Geometry: final body of the model. Coordinates: model frame, mm. Face numbers are marked on the shaded views. A direction names the side the tool comes from. Give positions to 0.01 mm unless a question says otherwise; leave off trailing zeros. Write each loop counter-clockwise with the first axis right and the second up, starting at its lowest first coordinate (ties: lowest second). Pieces come first, ordered by that corner, then holes. Notation, with made-up numbers: (9, 13.5) -> (36, 13.5) arc R30 cw to (36, 50.5) -> close; hole circle Ø5 at (77, 6). An arc over 180 degrees is marked (long way). Answer as a JSON object with one key per item and string values.
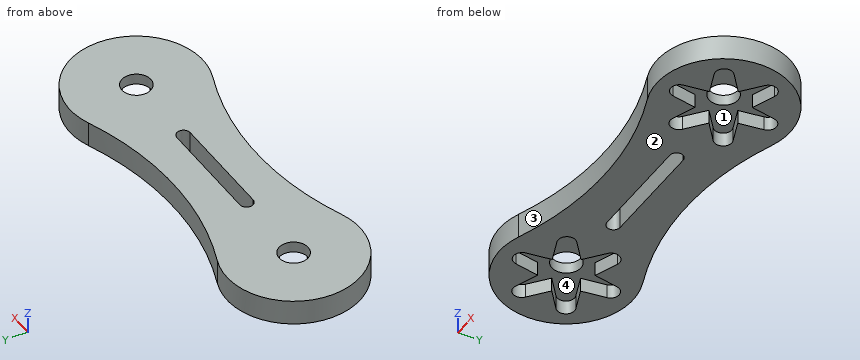
Autodesk Inventor part; units mm, degrees
ref_plane "Work Plane2" through (-40, 0, 7.55) normal (-1, 0, 0) x (0, -1, 0)
ref_plane "YZ Plane" through (0, 0, 0) normal (1, 0, 0) x (0, 1, 0)
ref_plane "XZ Plane" through (0, 0, 0) normal (0, 1, 0) x (-1, 0, 0)
sketch "Sketch1" plane through (0, 0, 0) normal (0, 0, 1) x (1, 0, 0)
  arc A0 (-72.7273, 18.6308) -> (-72.7273, -18.6308) centre (-80, 0) ccw
  arc A1 (-7.2727, -18.6308) -> (-72.7273, -18.6308) centre (-40, -102.4695) ccw
  arc A2 (-7.2727, -18.6308) -> (-7.2727, 18.6308) centre (0, 0) ccw
  arc A3 (-72.7273, 18.6308) -> (-7.2727, 18.6308) centre (-40, 102.4695) ccw
  arc A4 (-79.5765, 3.9775) -> (-79.5765, -3.9775) centre (-80, 0) ccw
  arc A5 (-0.4235, -3.9775) -> (-0.4235, 3.9775) centre (0, 0) ccw
  arc A6 (-80.4235, -3.9775) -> (-80.4235, 3.9775) centre (-80, 0) ccw
  arc A7 (-0.4235, 3.9775) -> (-0.4235, -3.9775) centre (0, 0) ccw
  point P0 (-103.8261, -115.9088)
  dimension "d0" = 20
  dimension "d1" = 20
  dimension "d2" = 90
  dimension "d3" = 90
  dimension "d4" = 4
  dimension "d7" = 80
  dimension "d33" = 4
extrude "Extrusion1" add sketch "Sketch1" along normal blind 7.55 contours A3 A2 A1 A0 | A6 A4 | A7 A5
sketch "Sketch3" plane through (0, 0, 7.55) normal (0, 0, 1) x (1, 0, 0)
  arc A0 (-72.7273, 18.6308) -> (-72.7273, -18.6308) centre (-80, 0) ccw
  arc A1 (-7.2727, -18.6308) -> (-72.7273, -18.6308) centre (-40, -102.4695) ccw
  arc A2 (-7.2727, -18.6308) -> (-7.2727, 18.6308) centre (0, 0) ccw
  arc A3 (-72.7273, 18.6308) -> (-7.2727, 18.6308) centre (-40, 102.4695) ccw
  line L0 (-56.02, 2) -> (-23.98, 2)
  line L1 (-56.02, -2) -> (-23.98, -2)
  arc A4 (-56.02, 2) -> (-56.02, -2) centre (-56.02, 0) ccw
  arc A5 (-23.98, -2) -> (-23.98, 2) centre (-23.98, 0) ccw
  point P0 (-83.48, 0)
  dimension "d12" = 2
extrude "Extrusion2" cut sketch "Sketch3" against normal blind 10 contours L0 A5 L1 A4
ref_plane "Work Plane2" through (-40, 0, 7.55) normal (-1, 0, 0) x (0, -1, 0)
ref_plane "Work Plane1" through (-100, 0, 7.55) normal (-1, 0, 0) x (0, -1, 0)
sketch "Sketch10" plane through (0, 0, 0) normal (0, 0, -1) x (-1, 0, 0)
  circle A0 centre (0, 0) radius 4.35
  dimension "d43" = 8.7
extrude "Extrusion7" cut sketch "Sketch10" against normal blind 10
mirror "Mirror4" about plane through (-40, 0, 7.55) normal (-1, 0, 0) of "Extrusion7"
sketch "Sketch9" plane through (0, 0, 0) normal (0, 0, -1) x (-1, 0, 0)
  arc A0 (13.113, 4.6066) -> (10.5459, 9.0529) centre (11.4723, 6.6235) ccw
  arc A1 (2.5671, 13.6595) -> (-2.5671, 13.6595) centre (0, 13.2471) ccw
  line L0 (13.113, 4.6066) -> (7.45, 0)
  line L1 (10.5459, 9.0529) -> (3.725, 6.4519)
  line L2 (3.725, 6.4519) -> (2.5671, 13.6595)
  line L3 (-2.5671, 13.6595) -> (-3.725, 6.4519)
  line L4 (-3.725, 6.4519) -> (-10.5459, 9.0529)
  line L5 (-13.113, 4.6066) -> (-7.45, 0)
  arc A2 (-10.5459, 9.0529) -> (-13.113, 4.6066) centre (-11.4723, 6.6235) ccw
  arc A3 (72.7273, -18.6308) -> (72.7273, 18.6308) centre (80, 0) ccw
  arc A4 (7.2727, 18.6308) -> (72.7273, 18.6308) centre (40, 102.4695) ccw
  arc A5 (7.2727, 18.6308) -> (7.2727, -18.6308) centre (0, 0) ccw
  arc A6 (72.7273, -18.6308) -> (7.2727, -18.6308) centre (40, -102.4695) ccw
  circle A7 centre (0, 0) radius 7.45 construction
  line L6 (-7.45, 0) -> (7.45, 0) construction
  arc A8 (10.5459, -9.0529) -> (13.113, -4.6066) centre (11.4723, -6.6235) ccw
  arc A9 (-2.5671, -13.6595) -> (2.5671, -13.6595) centre (0, -13.2471) ccw
  line L7 (13.113, -4.6066) -> (7.45, 0)
  line L8 (10.5459, -9.0529) -> (3.725, -6.4519)
  line L9 (3.725, -6.4519) -> (2.5671, -13.6595)
  line L10 (-2.5671, -13.6595) -> (-3.725, -6.4519)
  line L11 (-3.725, -6.4519) -> (-10.5459, -9.0529)
  line L12 (-13.113, -4.6066) -> (-7.45, 0)
  arc A10 (-13.113, -4.6066) -> (-10.5459, -9.0529) centre (-11.4723, -6.6235) ccw
  circle A11 centre (0, 0) radius 4.35
  dimension "diametro_petalo" = 2.6
  dimension "diametro_aspa" = 14.9
  dimension "largo_petalo" = 7.3
  dimension "d52" = 60
  dimension "d53" = 8.7
extrude "Extrusion8" cut sketch "Sketch9" against normal blind 4.25 contours L0 L7 A8 L8 L9 A9 L10 L11 A10 L12 L5 A2 L4 L3 A1 L2 L1 A0
mirror "Mirror5" about plane through (-40, 0, 7.55) normal (-1, 0, 0) of "Extrusion8"
equation "\"d0\" = radio_muslo"
equation "\"d1\" = d0"
equation "\"d2\" = curva"
equation "\"d3\" = d2"
equation "\"d4\" = 0.5 * diametro_servo"
equation "\"d7\" = distancia_centros"
equation "\"d33\" = d4"
equation "\"curva\" = 90"
equation "\"distancia_centros\" = 80"
equation "\"espesor\" = 3.3"
equation "\"diametro_servo\" = 8"
properties part number "Pata - Antebrazo" material "ABS Plastic"
Q1. Set-up query: the marked faces 3 and 4. Return all of +Z, -Z, +X, -X, +Y, -Y with unobstructed straight access to the full face (end or side cutting, diameter ignored); none if empty.
Values:
{"face 3": "+Z, -Z, -Y", "face 4": "-Z"}
Q2. Cut plane C-C (z = 6.25). Return the cut outline in (x, y), and give its area (3 significant figures).
Values:
{"outline": "(-72.73, -18.63) arc R90 cw to (-7.27, -18.63) arc R20 ccw (long way) to (-7.27, 18.63) arc R90 cw to (-72.73, 18.63) arc R20 ccw (long way) to start; hole circle Ø8.7 at (-80, 0); hole (-56.02, -2) -> (-23.98, -2) arc R2 ccw to (-23.98, 2) -> (-56.02, 2) arc R2 ccw to start; hole circle Ø8.7 at (0, 0)", "area": "3,460 mm²"}
Q3. Cut plane B-B (y = 17). Return the cut outline in (x, z), and give its area (3 significant figures).
Values:
{"outline": "(-90.54, 0) -> (-68.2, 0) -> (-68.2, 7.55) -> (-90.54, 7.55) -> close; (-11.8, 0) -> (10.54, 0) -> (10.54, 7.55) -> (-11.8, 7.55) -> close", "area": "337 mm²"}
Q4. Cut plane A-A (x = 0). Return the cut outline in (y, z).
Values:
{"outline": "(-20, 0) -> (-15.85, 0) -> (-15.85, 4.25) -> (-4.35, 4.25) -> (-4.35, 7.55) -> (-20, 7.55) -> close; (4.35, 4.25) -> (15.85, 4.25) -> (15.85, 0) -> (20, 0) -> (20, 7.55) -> (4.35, 7.55) -> close"}
Q5. First-contact query: P1, Ø1, axis at y = -9, z = 2.5, coming from the -X side; P2, Ø4, axis at x = -40.5, z = 2.5, coming from the -Y side; P3, Ø3, axis at y = 7, z = 5, coming from the -X side. Flat tips, straight axial feed; report the tip coordinate or a pass-through.
Values:
{"P1": "x = -98.1", "P2": "y = -12.5", "P3": "x = -99.23"}
Q6. Mould query, pull axis X, two halves, no side actions, for the marked faces 1 and 2. Classes: pulls with the +X half, pulls with the -X half, needs draft (parallel to the pull), parting line crosses it, or undercut.
Values:
{"face 1": "undercut", "face 2": "needs draft"}
Q7. Material intervals for L1, parallel to Y at x = 0, z = 6.35; L2, parallel to Y at x = -69, z = 3.75; L3, parallel to X at y = -3.5, z = 1.5, sorted ascending. Write a range as from..to.
Values:
{"L1": "-20..-4.35, 4.35..20", "L2": "-17.27..-9.18, -2.89..2.89, 9.18..17.27", "L3": "-99.69..-91.75, -68.25..-11.75, 11.75..19.69"}
Q8. Cut plane D-D (x = -74). Return the cut outline in (y, z).
Values:
{"outline": "(-19.08, 0) -> (-7.32, 0) -> (-7.32, 4.25) -> (7.32, 4.25) -> (7.32, 0) -> (19.08, 0) -> (19.08, 7.55) -> (-19.08, 7.55) -> close"}
